Geometry: final body of the model. Coordinates: model frame, mm. A direction names the side the tool comes from. Coordinates: 2 decimals unless noted, no trailing zeros. Loops run counter-clockwise (first coordinate to the right, second up) from the corner with the lowest first, then second, coordinate; pieces in that order, holes last. Notation, with made-up numbers: M 87.25,-13 L 137.25,-13 A6 cw 137.25,-9 Z; hole C 26,-10.75 d2. An arc over 180 degrees is marked long. Write each question's results on one line, items separated by ' | '. Start each with the question number.
from build123d import *

# Parameters (mm, degrees)
ESQUISSE1_R        = 1.5
BOSS_EXTRU_1_DEPTH = 6


with BuildPart() as part:
    # Esquisse1 → Boss.-Extru.1 (new body)
    with BuildSketch(Plane.XY):
        with BuildLine():
            Line((0, 18), (2.153216979, 21.894375))
            ThreePointArc((2.153216979, 21.894375), (6.098122971, 21.137949197), (9.83974396, 19.676875738))
            Line((9.83974396, 19.676875738), (9.606453592, 15.222222222))
            ThreePointArc((9.606453592, 15.222222222), (12.975935252, 12.474979132), (15.588457268, 9))
            Line((15.588457268, 9), (20.03769344, 9.082446896))
            ThreePointArc((20.03769344, 9.082446896), (21.355062473, 5.28784519), (21.960546236, 1.316969633))
            Line((21.960546236, 1.316969633), (17.986057943, -0.70832174))
            ThreePointArc((17.986057943, -0.70832174), (17.291616466, -5), (15.588457268, -9))
            Line((15.588457268, -9), (17.88447646, -12.811928104))
            ThreePointArc((17.88447646, -12.811928104), (15.256939503, -15.850104006), (12.120802276, -18.359906105))
            Line((12.120802276, -18.359906105), (8.37960435, -15.930543962))
            ThreePointArc((8.37960435, -15.930543962), (4.315681214, -17.474979132), (0, -18))
            Line((0, -18), (-2.153216979, -21.894375))
            ThreePointArc((-2.153216979, -21.894375), (-6.098122971, -21.137949197), (-9.83974396, -19.676875738))
            Line((-9.83974396, -19.676875738), (-9.606453592, -15.222222222))
            ThreePointArc((-9.606453592, -15.222222222), (-12.975935252, -12.474979132), (-15.588457268, -9))
            Line((-15.588457268, -9), (-20.03769344, -9.082446896))
            ThreePointArc((-20.03769344, -9.082446896), (-21.355062473, -5.28784519), (-21.960546236, -1.316969633))
            Line((-21.960546236, -1.316969633), (-17.986057943, 0.70832174))
            ThreePointArc((-17.986057943, 0.70832174), (-17.291616466, 5), (-15.588457268, 9))
            Line((-15.588457268, 9), (-17.88447646, 12.811928104))
            ThreePointArc((-17.88447646, 12.811928104), (-15.256939503, 15.850104006), (-12.120802276, 18.359906105))
            Line((-12.120802276, 18.359906105), (-8.37960435, 15.930543962))
            ThreePointArc((-8.37960435, 15.930543962), (-4.315681214, 17.474979132), (0, 18))
        make_face()
        with Locations((-10.743337321, 11.17276614)):
            Circle(ESQUISSE1_R, mode=Mode.SUBTRACT)
        with Locations((15.047567968, 3.717619972)):
            Circle(ESQUISSE1_R, mode=Mode.SUBTRACT)
        with Locations((-4.304230647, -14.890386111)):
            Circle(ESQUISSE1_R, mode=Mode.SUBTRACT)
        with BuildLine():
            ThreePointArc((-11.633900603, 7.787962299), (-13.591351713, -3.357850297), (-6.668605179, -12.309740248))
            ThreePointArc((-6.668605179, -12.309740248), (-3.332307598, -11.52804086), (-0.927622893, -13.969234616))
            ThreePointArc((-0.927622893, -13.969234616), (9.703659516, -10.091530707), (13.994850358, 0.379688631))
            ThreePointArc((13.994850358, 0.379688631), (11.64973004, 2.878157397), (12.561523496, 6.181272318))
            ThreePointArc((12.561523496, 6.181272318), (3.887692197, 13.449381004), (-7.326245179, 11.930051617))
            ThreePointArc((-7.326245179, 11.930051617), (-8.317422442, 8.649883463), (-11.633900603, 7.787962299))
        make_face(mode=Mode.SUBTRACT)
    extrude(amount=BOSS_EXTRU_1_DEPTH)


solid = part.part
Item 1: Ray query, L1, parallel to Y at x = -9.5, z = 4.7; L2, parallel to X at y = 11, z = 4.85; L3, parallel to X at y = 4.5, z = 3.3. Return the intervals inside material, ascending. Write a range as [from, to].
Item 2: Section B-B, the plane y = 16.5. Return loops of the section in (x, z), plus the area to 3 significant figures.
Item 3: Section A-A, the plane x = 0.5. Return loops of the section in (y, z), plus the area to 3 significant figures.
Item 4: Section C-C, the plane z = 4.4. Count the separate pieces of the cut face and the enclosed holes in it, plus the area to 3 significant figures.
Item 5: Set-up query: faces 1 (the flat face through (10.276, -17.162, 2.958)), 2 (the cylindrical face through (4.044, 13.403, 2.958)), 3 (the flat face through (-16.72, 10.88, 2.96)). Return all of +Z, -Z, +X, -X, +Y, -Y with unobstructed straight access to the full face (end or side cutting, diameter ignored); none if empty.
Item 6: Contact query for flat-ended pins moving along their axis: P1, Ø6, axis at x = 3.5, y = 13.5, coming from the +Z side; P2, Ø2.5, axis at x = -4.3, y = -14.89, coming from the +Z side. Output: stop coordinate, or through.
Item 7: Pull-direction query (Y, two-part tool) for faces 4 (the flat face through (-8, 10, 6)), 5 (the cylindrical face through (11.66, 2.83, 2.96)), 6 (the cylindrical face through (-21.341, -5.342, 2.958)), 7 (the cylindrical face through (-15.3, 15.81, 2.96)); classes: released by +Y, released by -Y, zero draft, split by the parting line, or undercut.
Solutions:
1) L1: y = [-19.84, -10.28], [7.9, 10.33], [12.01, 16.66] | L2: x = [-16.79, -12.23], [-9.25, -7.25], [8.66, 14.25] | L3: x = [-17.43, -13.26], [11.64, 13.77], [16.33, 21.53]
2) outline: M -14.55,0 L -9.26,0 L -9.26,6 L -14.55,6 Z; M -7.19,0 L 9.67,0 L 9.67,6 L -7.19,6 Z | area: 133 mm²
3) outline: M -17.99,0 L -13.99,0 L -13.99,6 L -17.99,6 Z; M 13.99,0 L 18.9,0 L 18.9,6 L 13.99,6 Z | area: 53.5 mm²
4) separate pieces: 1 | enclosed holes: 4 | area: 624 mm²
5) face 1: +Z, -Z, -Y | face 2: +Z, -Z | face 3: +Z, -Z, -X
6) P1: stops at z = 6 | P2: passes through
7) face 4: zero draft | face 5: undercut | face 6: released by -Y | face 7: released by +Y
